Read the model definition and answer for the solid it produces. Units are mm, in the model's axes. Coordinates: 2 decimals unless noted, no trailing zeros. Write each loop counter-clockwise with the first axis right and the second up, starting at its lowest first coordinate (ties: lowest second). Pieces come first, ordered by that corner, then holes.
(1) Find the intervals of material crossed by probe 1 along Y at (x, z) = (94, 1.7); probe 2 along X at (y, z) = (21, 0.4); probe 3 along X at (y, z) = (24, 1.85), in increasing order.
(2) Given pin 1 (1 mm diameter, centred on y = -2, z = 1.5, fed in from -X); pin 2 (1 mm diameter, centred on y = 43, z = 1.5, fed in from -X); pin 3 (1 mm diameter, centred on x = 88, z = 1.5, fed in from +Y); pin 4 (8 mm diameter, centred on x = 104, y = 7.5, fed in from -Z), each flat-ended and moving along its own axis, determine where each tip first touches the part or whether it passes through.
(3) Section B-B on y = 33 is taken. Write down the section's boundary in (x, z).
(4) Section D-D on y = 19 is taken. Write down the section's boundary in (x, z), then the cut area to 3 significant figures.
(5) Section C-C on x = 69 is taken. Write down the section's boundary in (y, z), then the cut area to 3 significant figures.
(6) Section A-A on y = 11.5 is taken. Write down the section's boundary in (x, z).
from build123d import *

# Parameters (mm, degrees)
SKETCH001_W   = 180
SKETCH001_H   = 60
SKETCH001_W_2 = 15
SKETCH001_H_2 = 3
SKETCH001_W_3 = 3
SKETCH001_H_3 = 15
PAD_DEPTH     = 2
SKETCH_R      = 1.75
SKETCH_R_2    = 26.5
SKETCH_W      = 14
SKETCH_H      = 9.5


with BuildPart() as part:
    # Sketch001 → Pad (new body)
    with BuildSketch(Plane.XY):
        with Locations((90, 30)):
            Rectangle(SKETCH001_W, SKETCH001_H)
        with Locations((36.5, 61.5)):
            Rectangle(SKETCH001_W_2, SKETCH001_H_2)
        with Locations((36.5, -1.5)):
            Rectangle(SKETCH001_W_2, SKETCH001_H_2)
        with Locations((143.5, 61.5)):
            Rectangle(SKETCH001_W_2, SKETCH001_H_2)
        with Locations((143.5, -1.5)):
            Rectangle(SKETCH001_W_2, SKETCH001_H_2)
        with Locations((-1.5, 30)):
            Rectangle(SKETCH001_W_3, SKETCH001_H_3)
        with Locations((181.5, 30)):
            Rectangle(SKETCH001_W_3, SKETCH001_H_3)
    extrude(amount=PAD_DEPTH)

    # Sketch → Groove (revolve, cut)
    with BuildSketch(Plane.XY):
        with Locations((14, 52.754121)):
            Circle(SKETCH_R)
        with Locations((59, 52.754121)):
            Circle(SKETCH_R)
        with Locations((14, 7.245879)):
            Circle(SKETCH_R)
        with Locations((59, 7.245879)):
            Circle(SKETCH_R)
        with Locations((36.5, 30)):
            Circle(SKETCH_R_2)
        with Locations((166, 52.754121)):
            Circle(SKETCH_R)
        with Locations((121, 52.754121)):
            Circle(SKETCH_R)
        with Locations((166, 7.245879)):
            Circle(SKETCH_R)
        with Locations((121, 7.245879)):
            Circle(SKETCH_R)
        with Locations((143.5, 30)):
            Circle(SKETCH_R_2)
        with Locations((90, 30)):
            Rectangle(SKETCH_W, SKETCH_H)
    revolve(axis=Axis((0, 0, 0), (0, 1, 0)), mode=Mode.SUBTRACT)


solid = part.part
Response:
1. probe 1: y = 0 to 25.25, 34.75 to 60
1. probe 2: x = 0 to 11.57, 61.42 to 118.57, 168.42 to 180
1. probe 3: x = -3 to 10.53, 62.28 to 117.67, 169.3 to 183
2. pin 1: stops at x = 29
2. pin 2: stops at x = 0
2. pin 3: stops at y = 60
2. pin 4: stops at z = 0
3. outline: (-3, 0) - (10.17, 0) arc R10.17 ccw to (9.97, 2) - (-3, 2) - close; (62.8, 2) arc R62.83 cw to (62.83, 0) - (83, 0) arc R83 ccw to (82.98, 2) - close; (96.98, 2) arc R97 cw to (97, 0) - (117.17, 0) arc R117.17 ccw to (117.15, 2) - close; (169.82, 2) arc R169.83 cw to (169.83, 0) - (183, 0) - (183, 2) - close
4. outline: (0, 0) - (12.39, 0) arc R12.39 ccw to (12.23, 2) - (0, 2) - close; (60.58, 2) arc R60.61 cw to (60.61, 0) - (119.39, 0) arc R119.39 ccw to (119.37, 2) - close; (167.6, 2) arc R167.61 cw to (167.61, 0) - (180, 0) - (180, 2) - close
4. area: 167 mm2
5. outline: (0, 0) - (60, 0) - (60, 2) - (0, 2) - close
5. area: 120 mm2
6. outline: (0, 0) - (17.53, 0) arc R17.53 ccw to (17.41, 2) - (0, 2) - close; (55.44, 2) arc R55.47 cw to (55.47, 0) - (124.53, 0) arc R124.53 ccw to (124.51, 2) - close; (162.46, 2) arc R162.47 cw to (162.47, 0) - (180, 0) - (180, 2) - close
